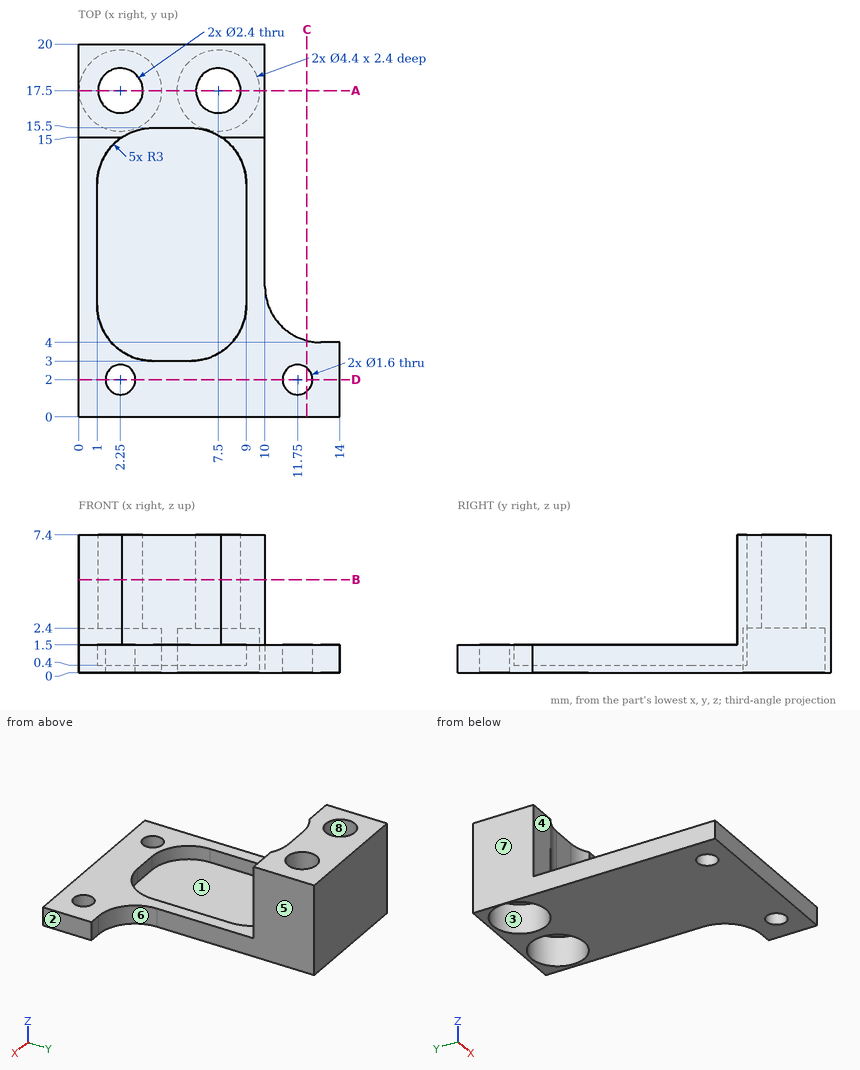
For this review, use the dimensioned drawing (mm, ordinates from the lowest corner) and the shaded views. A direction names the side the tool comes from. Coordinates: 2 decimals unless noted, no trailing zeros. Write each loop counter-clockwise with the first axis right and the second up, starting at its lowest first coordinate (ties: lowest second). Pieces come first, ordered by that corner, then holes. Notation, with made-up numbers: (40, 22.25) - (66, 22.25) arc R27 cw to (66, 55.25) - close; hole circle Ø1 at (87.25, -14.75). An arc over 180 degrees is marked (long way). Answer in a Markdown table with one row per item. Add a question column.
Q1. Consider section A-A on y = 17.5. Give the boundary of the cut face in (x, z), then the cut area to 3 significant figures.
Q2. For the marked faces 1, 2, 3, 4 and 5, list the 3-axis set-ups (+Z, -Z, +X, -X, +Y, -Y) from which the entire face can be reached by the end or side of a thin tool; tool diameter is ignored.
Q3. Consider section B-B on z = 5. Give the boundary of the cut face in (x, y), then the cut area to 3 significant figures.
Q4. Draft analysis for pull direction Y (two halves, no side actions). For the marked faces 6, 7 and 8, state which applies: +Y half, -Y half, draft (parallel to the pull), parting line (faces both ways), or undercut.
Q5. To check wall thickness, follow line 1 along Y through (x, z) = (6, 1); line 2 along Y through (x, z) = (2.25, 4.95); line 3 along Y through (x, z) = (7.5, 1.3). State the ranges of each line that lie inside material, in increasing order. Write a range as from..to.
Q6. Clearance check with flat-ended pins moving along their axes: pin 1 (0.8 mm diameter, centred on x = 13.5, z = 1, fed in from +Y); pin 2 (6.5 mm diameter, centred on x = 7, y = 10, fed in from +Z); pin 3 (0.9 mm diameter, centred on y = 9, z = 0.5, fed in from -X); pin 4 (3.5 mm diameter, centred on x = 2.25, y = 17.5, fed in from -Z). State where each tip first meets the part, or that it passes through.
Q7. Consider section D-D on y = 2. Give the boundary of the cut face in (x, z), then the cut area to 3 significant figures.
Q8. Consider section C-C on x = 12.25. Give the boundary of the cut face in (y, z).
Answers below:
| question | item | result |
|---|---|---|
| 1 | outline | (0, 0) - (0.05, 0) - (0.05, 2.4) - (1.05, 2.4) - (1.05, 7.4) - (0, 7.4) - close; (3.45, 2.4) - (4.45, 2.4) - (4.45, 0) - (5.3, 0) - (5.3, 2.4) - (6.3, 2.4) - (6.3, 7.4) - (3.45, 7.4) - close; (8.7, 2.4) - (9.7, 2.4) - (9.7, 0) - (10, 0) - (10, 7.4) - (8.7, 7.4) - close |
| 1 | area | 28.9 mm² |
| 2 | face 1 | +Z |
| 2 | face 2 | +Z, -Z, +X, +Y, -Y |
| 2 | face 3 | -Z |
| 2 | face 4 | +Z, +X, -X, -Y |
| 2 | face 5 | +Z, -Z, +X, +Y |
| 3 | outline | (0, 15) - (2.34, 15) arc R3 cw to (4, 15.5) - (6, 15.5) arc R3 cw to (7.66, 15) - (10, 15) - (10, 20) - (0, 20) - close; hole circle Ø2.4 at (2.25, 17.5); hole circle Ø2.4 at (7.5, 17.5) |
| 3 | area | 38.8 mm² |
| 4 | face 6 | +Y half |
| 4 | face 7 | draft |
| 4 | face 8 | undercut |
| 5 | line 1 | 0..3, 15.5..15.89, 19.11..20 |
| 5 | line 2 | 15..16.3, 18.7..20 |
| 5 | line 3 | 0..3.4, 15.1..15.3, 19.7..20 |
| 6 | pin 1 | y = 4 |
| 6 | pin 2 | z = 1.5 |
| 6 | pin 3 | x = 0 |
| 6 | pin 4 | z = 2.4 |
| 7 | outline | (0, 0) - (1.45, 0) - (1.45, 1.5) - (0, 1.5) - close; (3.05, 0) - (10.95, 0) - (10.95, 1.5) - (3.05, 1.5) - close; (12.55, 0) - (14, 0) - (14, 1.5) - (12.55, 1.5) - close |
| 7 | area | 16.2 mm² |
| 8 | outline | (0, 0) - (1.38, 0) - (1.38, 1.5) - (0, 1.5) - close; (2.62, 0) - (4.1, 0) - (4.1, 1.5) - (2.62, 1.5) - close |
